```python
from build123d import *

# Parameters (mm, degrees)
ESQUISSE1_W             = 410
ESQUISSE1_H             = 330
BOSS_EXTRU_1_DEPTH      = 5
ESQUISSE2_W             = 10
ESQUISSE2_H             = 5
ENL_V_MAT_EXTRU_1_DEPTH = 527.331644498


with BuildPart() as part:
    # Esquisse1 → Boss.-Extru.1 (new body)
    with BuildSketch(Plane.XY):
        with Locations((205, 165)):
            Rectangle(ESQUISSE1_W, ESQUISSE1_H)
    extrude(amount=BOSS_EXTRU_1_DEPTH)

    # Esquisse2 → Enlèv. mat.-Extru.1 (cut, through all)
    with BuildSketch(Plane.XY.offset(5)):
        with Locations((25, 2.5)):
            Rectangle(ESQUISSE2_W, ESQUISSE2_H)
        with Locations((5, 2.5)):
            Rectangle(ESQUISSE2_W, ESQUISSE2_H)
        with Locations((45, 2.5)):
            Rectangle(ESQUISSE2_W, ESQUISSE2_H)
        with Locations((65, 2.5)):
            Rectangle(ESQUISSE2_W, ESQUISSE2_H)
        with Locations((85, 2.5)):
            Rectangle(ESQUISSE2_W, ESQUISSE2_H)
        with Locations((105, 2.5)):
            Rectangle(ESQUISSE2_W, ESQUISSE2_H)
        with Locations((125, 2.5)):
            Rectangle(ESQUISSE2_W, ESQUISSE2_H)
        with Locations((145, 2.5)):
            Rectangle(ESQUISSE2_W, ESQUISSE2_H)
        with Locations((165, 2.5)):
            Rectangle(ESQUISSE2_W, ESQUISSE2_H)
        with Locations((185, 2.5)):
            Rectangle(ESQUISSE2_W, ESQUISSE2_H)
        with Locations((205, 2.5)):
            Rectangle(ESQUISSE2_W, ESQUISSE2_H)
        with Locations((225, 2.5)):
            Rectangle(ESQUISSE2_W, ESQUISSE2_H)
        with Locations((245, 2.5)):
            Rectangle(ESQUISSE2_W, ESQUISSE2_H)
        with Locations((265, 2.5)):
            Rectangle(ESQUISSE2_W, ESQUISSE2_H)
        with Locations((285, 2.5)):
            Rectangle(ESQUISSE2_W, ESQUISSE2_H)
        with Locations((305, 2.5)):
            Rectangle(ESQUISSE2_W, ESQUISSE2_H)
        with Locations((325, 2.5)):
            Rectangle(ESQUISSE2_W, ESQUISSE2_H)
        with Locations((345, 2.5)):
            Rectangle(ESQUISSE2_W, ESQUISSE2_H)
        with Locations((365, 2.5)):
            Rectangle(ESQUISSE2_W, ESQUISSE2_H)
        with Locations((385, 2.5)):
            Rectangle(ESQUISSE2_W, ESQUISSE2_H)
        with Locations((405, 2.5)):
            Rectangle(ESQUISSE2_W, ESQUISSE2_H)
    extrude(amount=-ENL_V_MAT_EXTRU_1_DEPTH, mode=Mode.SUBTRACT)


solid = part.part
```
Design review of the part built by this model. Coordinates are the model's own, in mm. Coordinates: 2 decimals unless noted, no trailing zeros. Order: outer loops, then holes, each group sorted by start corner. A loop starts at its lowest first (then second) coordinate and runs counter-clockwise, first axis right, second up. Notation, with made-up numbers: (86, 74) -> (109, 74) arc R9 cw to (109, 90) -> close; hole circle Ø8 at (31.5, 28.5). An arc over 180 degrees is marked (long way). One line per item, written item: value. Start each with the question number.
Q1. For probe 1 along Y at (x, z) = (221, 1.5), list the stretches that pass through material, from the lowest coordinate up.
Q2. Insertion check: pin 1 Ø1.5 at (x, z) = (4.5, 1.5) entering from -Y; pin 2 Ø2.5 at (y, z) = (1.5, 3) entering from -X; pin 3 Ø2.5 at (y, z) = (3.5, 3) entering from +X. Each pin has a flat end and moves straight along its axis. Give the tip position at first contact, or say it passes through.
Q3. Take a section at A-A, the plane x = 225. State the section outline as (y, z) points, then the cut area to 4 significant figures.
Values follow:
1. probe 1: y = 5 to 330
2. pin 1: stops at y = 5
2. pin 2: stops at x = 10
2. pin 3: stops at x = 400
3. outline: (5, 0) -> (330, 0) -> (330, 5) -> (5, 5) -> close
3. area: 1,625 mm2
